Here's the drawing with two shaded views (mm, measured from the low corner). I have some questions. Round coordinates to 2 decimals unless told otherwise and drop trailing zeros. Loops run counter-clockwise (first coordinate to the right, second up) from the corner with the lowest first, then second, coordinate; pieces in that order, holes last. Notation, with made-up numbers: (15, 8) -> (22, 8) arc R16 ccw to (22, 35) -> close; hole circle Ø9 at (62.5, -9). An arc over 180 degrees is marked (long way). Write each question's results on one line, items separated by ' | '.
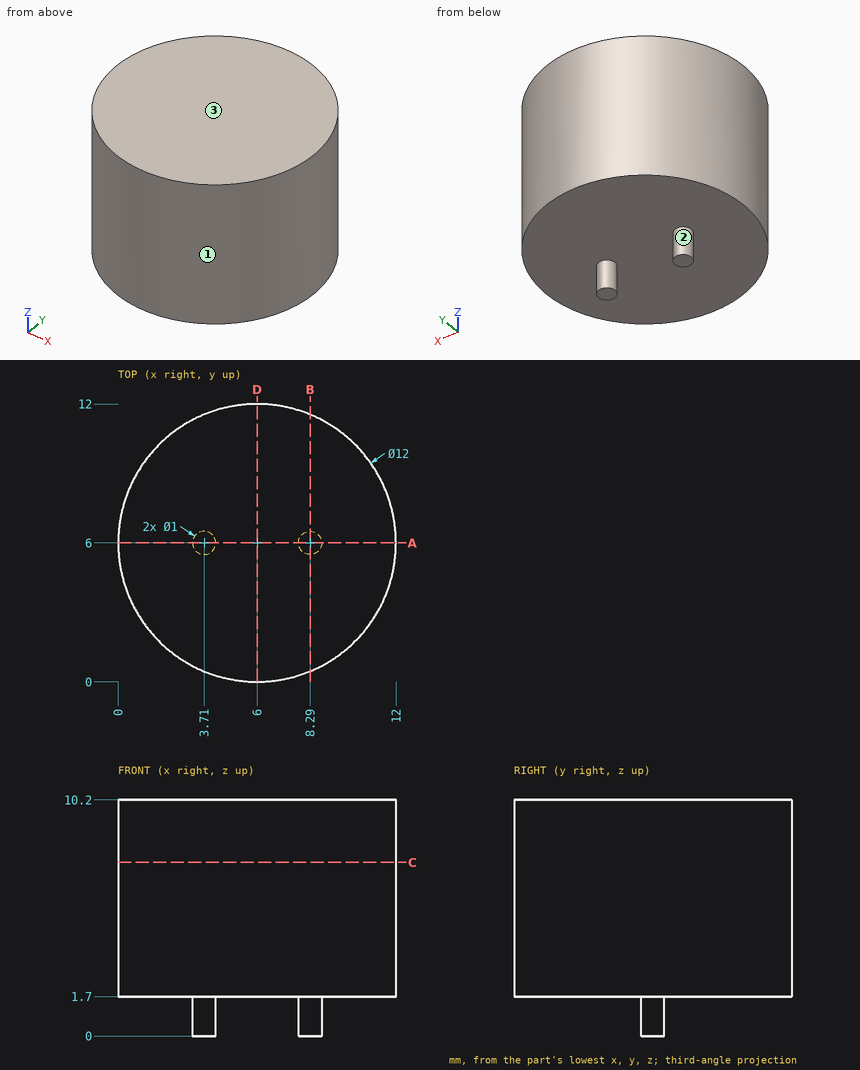
1. If we section it at B-B (x = 8.29): List the corners of the cut face in (y, z) for me, then the cut area to 3 significant figures.
Final values:
outline: (0.45, 1.7) -> (5.5, 1.7) -> (5.5, 0) -> (6.5, 0) -> (6.5, 1.7) -> (11.55, 1.7) -> (11.55, 10.2) -> (0.45, 10.2) -> close | area: 96.0 mm2
2. If we section it at D-D (x = 6): List the corners of the cut face in (y, z) for me, then the cut area to 3 significant figures.
Final values:
outline: (0, 1.7) -> (12, 1.7) -> (12, 10.2) -> (0, 10.2) -> close | area: 102 mm2
3. If we section it at A-A (y = 6): List the corners of the cut face in (x, z) for me, then the cut area to 3 significant figures.
Final values:
outline: (0, 1.7) -> (3.21, 1.7) -> (3.21, 0) -> (4.21, 0) -> (4.21, 1.7) -> (7.79, 1.7) -> (7.79, 0) -> (8.79, 0) -> (8.79, 1.7) -> (12, 1.7) -> (12, 10.2) -> (0, 10.2) -> close | area: 105 mm2
4. Please list where these lines run through material, in increasing order: line 1 (Z direction, x = 6.25, y = 7.5); line 2 (Y direction, x = 8.25, z = 1); line 3 (X direction, y = 8, z = 9.75). Write a range as from..to.
Final values:
line 1: 1.7..10.2 | line 2: 5.5..6.5 | line 3: 0.34..11.66
5. Will these pins go through, and if not, where does the flat tip stop? pin 1 (3 mm diameter, centred on x = 6.5, z = 3, fed in from +Y); pin 2 (4 mm diameter, centred on y = 3, z = 5, fed in from +X).
Final values:
pin 1: y = 12 | pin 2: x = 11.92
6. We'd pull the mould along X, two halves only. Please class the marked faces 1, 2 and 3: pulls with the +X half, pulls with the -X half, needs draft (parallel to the pull), parting line crosses it, or undercut.
Final values:
face 1: parting line crosses it | face 2: undercut | face 3: needs draft
7. If we section it at C-C (z = 7.5): List the corners of the cut face in (x, y) for me.
Final values:
outline: circle Ø12 at (6, 6)
